Part print with two shaded views. Sizes in mm from the minimum x, y, z corner. A direction names the side the tool comes from. Round coordinates to 2 decimals unless told otherwise and drop trailing zeros. Write each loop counter-clockwise with the first axis right and the second up, starting at its lowest first coordinate (ties: lowest second). Pieces come first, ordered by that corner, then holes. Notation, with made-up numbers: (20.25, 89) - (52.25, 89) arc R31 cw to (52.25, 124) - close; hole circle Ø2 at (16, -34). An arc over 180 degrees is marked (long way). Use one line per item in the form item = value. Start each with the question number.
Item 1: Band-saw the part on B-B, the plane y = 737. List the corners of the cut face in (x, z), and give its area (3 significant figures).
Item 2: Tool access for the marked faces 1 and 2: list every direction of +Z, -Z, +X, -X, +Y, -Y with a clear straight run to the whole face (end or side of a thin tool).
Item 3: Pin check, flat tips, straight feed: pin 1 (10 mm diameter, centred on y = 213.5, z = 24, fed in from +X); pin 2 (25 mm diameter, centred on x = 77, y = 368, fed in from +Z); pin 3 (20.5 mm diameter, centred on y = 306.5, z = 28, fed in from -X). Stop position of each tip, or through.
Item 4: Band-saw the part on A-A, the plane z = 24. List the corners of the cut face in (x, y).
Item 5: Drill centre lines: L1, parallel to X at y = 890, z = 28; L2, parallel to X at y = 636.5, z = 47; L3, parallel to Z at x = 150.5, y = 63.5. Where is each one in solid material? Low to high.
Item 6: Band-saw the part on C-C, the plane x = 18.5. List the corners of the cut face in (y, z), and give its area (3 significant figures).
Item 7: Band-saw the part on D-D, the plane x = 76. List the corners of the cut face in (y, z).
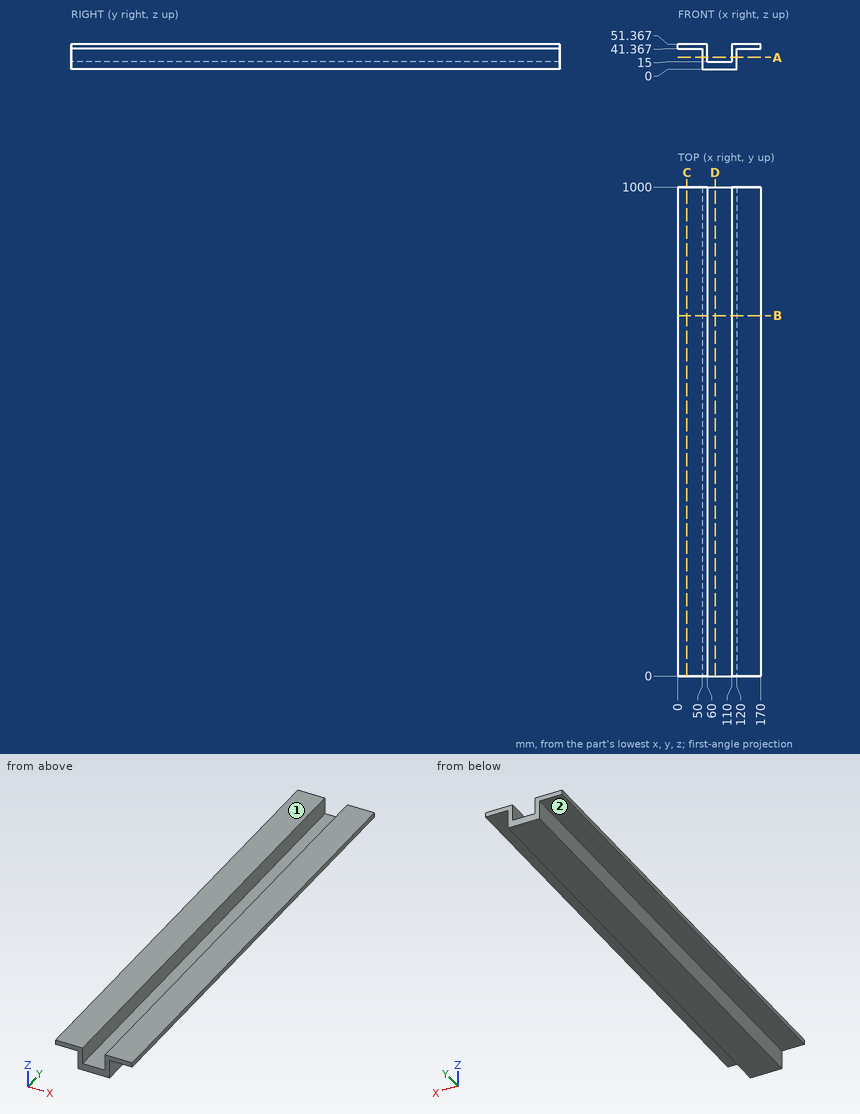
Determined:
q1.outline = (0, 41.37) - (50, 41.37) - (50, 0) - (120, 0) - (120, 41.37) - (170, 41.37) - (170, 51.37) - (110, 51.37) - (110, 15) - (60, 15) - (60, 51.37) - (0, 51.37) - close
q1.area = 2,780 mm²
q2.face_1 = +Z, +X, -X, +Y, -Y
q2.face_2 = -Z, -X, +Y, -Y
q3.pin_1 = 120
q3.pin_2 = 15
q3.pin_3 = 50
q4.outline = (50, 0) - (60, 0) - (60, 1000) - (50, 1000) - close; (110, 0) - (120, 0) - (120, 1000) - (110, 1000) - close
q5.L1 = 50 to 60, 110 to 120
q5.L2 = 0 to 60, 110 to 170
q5.L3 = 41.37 to 51.37
q6.outline = (0, 41.37) - (1000, 41.37) - (1000, 51.37) - (0, 51.37) - close
q6.area = 10,000 mm²
q7.outline = (0, 0) - (1000, 0) - (1000, 15) - (0, 15) - close
